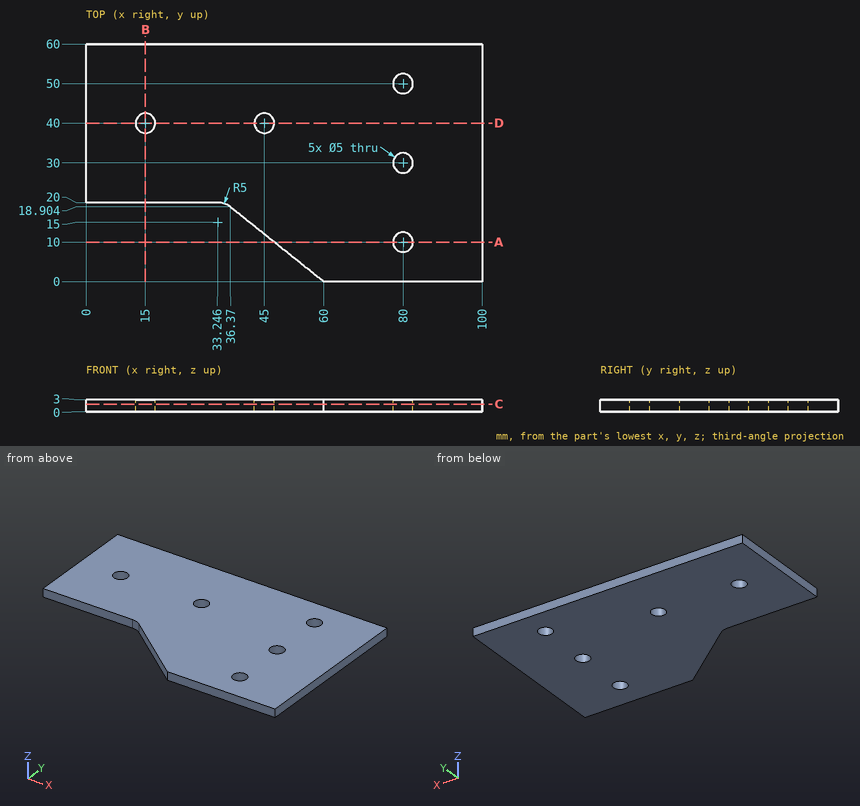
Geometry: see drawing. Coordinates: mm, zero at the bounding-box minimum. Round coordinates to 2 decimals unless told otherwise and drop trailing zeros. Loops run counter-clockwise (first coordinate to the right, second up) from the corner with the lowest first, then second, coordinate; pieces in that order, holes last. Notation, with made-up numbers: M 16,-6 L 75,-6 A25 cw 75,20 Z; hole C -17,85.5 d7. An arc over 180 degrees is marked long. Use a Markdown table: item, result. Add a question column.
1. Cut plane B-B, the plane x = 15. Output: boundary loops of the cut face in (y, z).
2. Ray query, line 1 along Y through (x, z) = (80, 2.1); line 2 along X through (y, z) = (30, 1.4); line 3 along Y through (x, z) = (78.5, 0.4). Return the intervals inside material, ascending. Write a range as [from, to].
3. Contact query for a flat-ended pin moving along its axis: pin 1 (3 mm diameter, centred on x = 80, y = 10, fed in from +Z). Output: stop coordinate, or through.
4. Cut plane A-A, the plane y = 10. Output: boundary loops of the cut face in (x, z).
5. Cut plane C-C, the plane z = 1.9. Output: boundary loops of the cut face in (x, y) (1 decimal), and give its area (3 significant figures).
6. Cut plane D-D, the plane y = 40. Output: boundary loops of the cut face in (x, z), and give its area (3 significant figures).
Solution:
| question | item | result |
|---|---|---|
| 1 | outline | M 20,0 L 37.5,0 L 37.5,3 L 20,3 Z; M 42.5,0 L 60,0 L 60,3 L 42.5,3 Z |
| 2 | line 1 | y = [0, 7.5], [12.5, 27.5], [32.5, 47.5], [52.5, 60] |
| 2 | line 2 | x = [0, 77.5], [82.5, 100] |
| 2 | line 3 | y = [0, 8], [12, 28], [32, 48], [52, 60] |
| 3 | pin 1 | passes through |
| 4 | outline | M 47.5,0 L 77.5,0 L 77.5,3 L 47.5,3 Z; M 82.5,0 L 100,0 L 100,3 L 82.5,3 Z |
| 5 | outline | M 0,20 L 33.2,20 A5 cw 36.4,18.9 L 60,0 L 100,0 L 100,60 L 0,60 Z; hole C 15,40 d5; hole C 45,40 d5; hole C 80,10 d5; hole C 80,30 d5; hole C 80,50 d5 |
| 5 | area | 4,950 mm2 |
| 6 | outline | M 0,0 L 12.5,0 L 12.5,3 L 0,3 Z; M 17.5,0 L 42.5,0 L 42.5,3 L 17.5,3 Z; M 47.5,0 L 100,0 L 100,3 L 47.5,3 Z |
| 6 | area | 270 mm2 |
